Here's the drawing with two shaded views (mm, measured from the low corner). I have some questions. A direction names the side the tool comes from. Round coordinates to 2 decimals unless told otherwise and drop trailing zeros. Order: outer loops, then holes, each group sorted by start corner. A loop starts at its lowest first (then second) coordinate and runs counter-clockwise, first axis right, second up. Notation, with made-up numbers: M 84,79 L 119,79 A33 cw 119,114 Z; hole C 70.5,62 d3. An arc over 180 degrees is marked long. One line per question, with ' | ' between items.
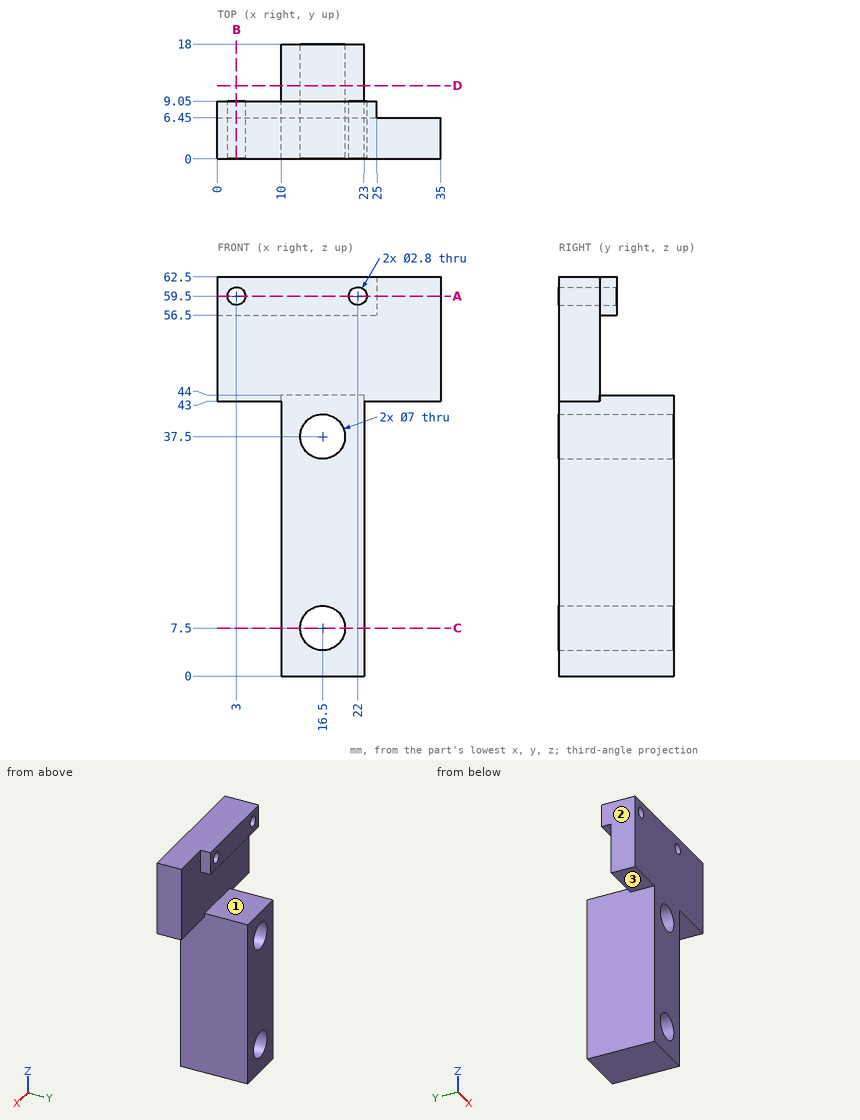
(1) On a 3-axis mill with a long thin cutter (end or side, diameter ignored), from which of +Z, -Z, +X, -X, +Y, -Y can I reach the whole of each face in a straight line? I mean the marked faces 1, 2 and 3. Say none if no direction works.
Final values:
face 1: +X, -X, +Y | face 2: +Z, -Z, -X, +Y, -Y | face 3: -Z, -X, +Y, -Y
(2) Please list where these lines run through material, in increasing order: probe 1 along Z at (x, y) = (16.5, 7); probe 2 along Z at (x, y) = (16.5, 9.75); probe 3 along X at (y, z) = (13, 7.5). Write a range as [from, to].
Final values:
probe 1: [0, 4], [11, 34], [41, 44], [56.5, 62.5] | probe 2: [0, 4], [11, 34], [41, 44] | probe 3: [10, 13], [20, 23]
(3) If we section it at D-D on y = 11.5: Please give me the cut outline in (x, z), plus the area to 3 significant figures.
Final values:
outline: M 10,0 L 23,0 L 23,44 L 10,44 Z; hole C 16.5,7.5 d7; hole C 16.5,37.5 d7 | area: 495 mm^2
(4) If we section it at B-B on x = 3: Please give me the cut outline in (y, z), plus the area to 3 significant figures.
Final values:
outline: M 0,43 L 6.45,43 L 6.45,56.5 L 9.05,56.5 L 9.05,58.1 L 0,58.1 Z; M 0,60.9 L 9.05,60.9 L 9.05,62.5 L 0,62.5 Z | area: 116 mm^2
(5) If we section it at C-C on z = 7.5: Please give me the cut outline in (x, y), plus the area to 3 significant figures.
Final values:
outline: M 10,0 L 13,0 L 13,18 L 10,18 Z; M 20,0 L 23,0 L 23,18 L 20,18 Z | area: 108 mm^2
(6) If we section it at A-A on z = 59.5: Please give me the cut outline in (x, y).
Final values:
outline: M 0,0 L 1.6,0 L 1.6,9.05 L 0,9.05 Z; M 4.4,0 L 20.6,0 L 20.6,9.05 L 4.4,9.05 Z; M 23.4,0 L 35,0 L 35,6.45 L 25,6.45 L 25,9.05 L 23.4,9.05 Z
(7) Will these pins go through, and if not, where does the flat tip stop? pin 1 Ø3.5 at (x, y) = (14, 12) entering from +Z; pin 2 Ø5 at (x, y) = (7, 2.5) entering from -Z; pin 3 Ø6.5 at (x, z) = (6.5, 59.5) entering from +Y.
Final values:
pin 1: z = 44 | pin 2: z = 43 | pin 3: y = 9.05
